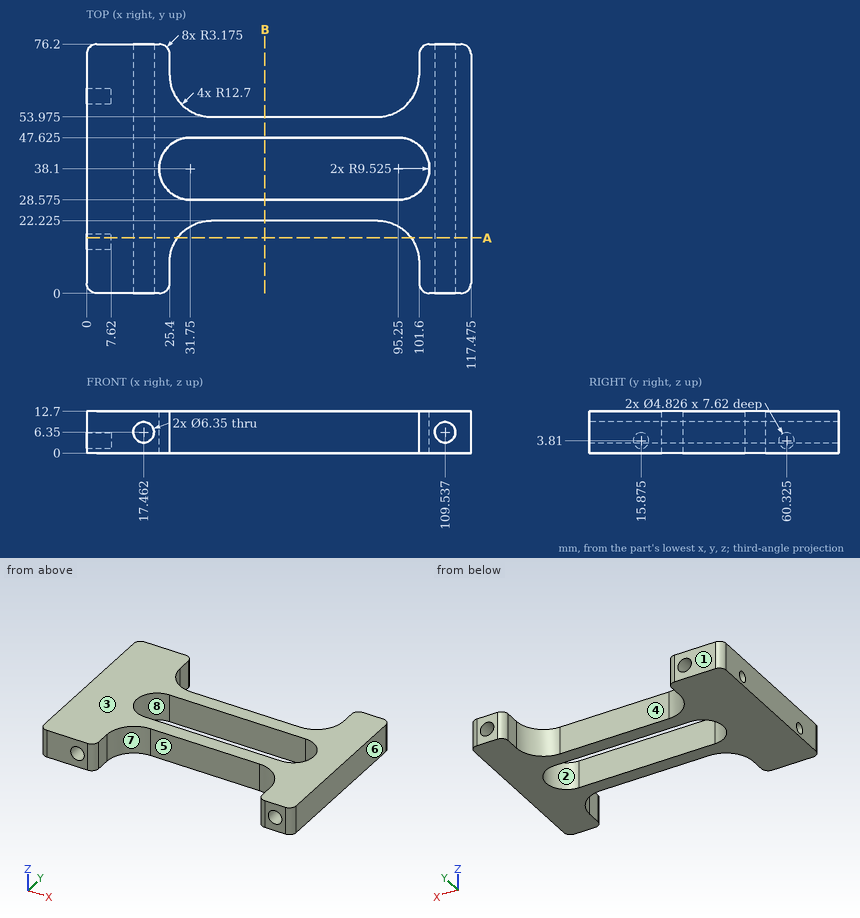
Print and shaded views of the part. All mm, measured from the part's lowest x, y and z. A direction names the side the tool comes from. Give positions to 0.01 mm unless a question says otherwise; leave off trailing zeros. Write each loop counter-clockwise with the first axis right and the second up, starting at its lowest first coordinate (ties: lowest second). Pieces come first, ordered by that corner, then holes. Notation, with made-up numbers: (77, -34) -> (97, -34) arc R12 ccw to (97, -26) -> close; hole circle Ø6 at (12, 51.25). An arc over 180 degrees is marked (long way). Use CSV: the item, a comma, the result in double quotes. Start each with the question number.
1) Cut at A-A on y = 17. Count the separate pieces of the cut face and the enclosed holes in it, plus the area to 3 significant figures.
2) Drill centre lines: L1, parallel to X at y = 67.5, z = 6.5 (1 decimal); L2, parallel to Y at x = 3.5, z = 3.81; L3, parallel to X at y = 24, z = 6.5 (1 decimal). Where is each one in solid material? Low to high.
3) Two-plate mould, pull along Y, no slides. Class the marked faces 6, 7 and 8: released by +Y, released by -Y, zero draft, split by the parting line, or undercut.
4) Tool access for the marked faces 1, 2, 3, 4 and 5: list every direction of +Z, -Z, +X, -X, +Y, -Y with a clear straight run to the whole face (end or side of a thin tool).
5) Cut at B-B on x = 54.5. List the corners of the cut face in (y, z) (1 decimal), plus the area to 3 significant figures.
6) Pin check, flat tips, straight feed: P1, Ø5.5, axis at x = 17.46, z = 6.35, coming from the +Y side; P2, Ø6.5, axis at x = 61.5, z = 9, coming from the -Y side (1 decimal); P3, Ø4, axis at x = 70, z = 8.5, coming from the +Y side (1 decimal); P4, Ø6, axis at x = 96, z = 5.5, coming from the -Y side (1 decimal). Stop position of each tip, or through.
Final values:
1,separate pieces,"2"
1,enclosed holes,"2"
1,area,"490 mm2"
2,L1,"x = 0 to 14.3, 20.6 to 25.4, 101.6 to 106.4, 112.7 to 117.5"
2,L2,"y = 0 to 13.46, 18.29 to 57.91, 62.74 to 76.2"
2,L3,"x = 0 to 14.3, 20.6 to 106.4, 112.7 to 117.5"
3,face 6,"zero draft"
3,face 7,"released by -Y"
3,face 8,"undercut"
4,face 1,"+Z, -Z, +X, -X, +Y"
4,face 2,"+Z, -Z"
4,face 3,"+Z, +X, -X, +Y, -Y"
4,face 4,"+Z, -Z, +Y"
4,face 5,"+Z, -Z, -Y"
5,outline,"(22.2, 0) -> (28.6, 0) -> (28.6, 12.7) -> (22.2, 12.7) -> close; (47.6, 0) -> (54, 0) -> (54, 12.7) -> (47.6, 12.7) -> close"
5,area,"161 mm2"
6,P1,"passes through"
6,P2,"stops at y = 22.2"
6,P3,"stops at y = 54"
6,P4,"stops at y = 17.2"
